from build123d import *

# Parameters (mm, degrees)
F0_R           = 50.8
F1_DEPTH       = 6.35
F3_R           = 25.4
F1_FACE_R      = 50.8
F6_D           = 17.4625
F6_CBORE_D     = 30.1625
F6_CBORE_DEPTH = 19.05


with BuildPart() as f1:
    # F0 (on Top) → F1 (new body)
    with BuildSketch(Plane.XY):
        Circle(F0_R)
    extrude(amount=F1_DEPTH)

    # F3 (on offset) → F4 section 0
    with BuildSketch(Plane.XY.offset(25.4)):
        Circle(F3_R)
    # F1_face (on face) → F4 section 1
    with BuildSketch(Plane.XY.offset(6.35)):
        Circle(F1_FACE_R)
    loft()

    # F6 (through all)
    with Locations(Plane(origin=(0, 0, 0), x_dir=(1, 0, 0), z_dir=(0, 0, -1))):
        with Locations((0, 0)):
            CounterBoreHole(F6_D / 2, F6_CBORE_D / 2, F6_CBORE_DEPTH)


solid = f1.part
CAD build for the part. Positions are in the model's coordinates, mm. A direction names the side the tool comes from. Coordinates: 2 decimals unless noted, no trailing zeros. Loops run counter-clockwise (first coordinate to the right, second up) from the corner with the lowest first, then second, coordinate; pieces in that order, holes last. Notation, with made-up numbers: (62, -3.75) - (89, -3.75) arc R34 cw to (89, 33.25) - close; hole circle Ø3 at (-13.5, -34). An arc over 180 degrees is marked (long way). Write item = value, one per line. Start each with the question number.
Q1. Cut at A-A, the plane x = 0. List the corners of the cut face in (y, z), then the cut area to 3 significant figures.
Q2. Drill centre lines: L1, parallel to Y at x = 0, z = 4.5; L2, parallel to Y at x = 9, z = 12.5; L3, parallel to X at y = -6, z = 24. Where is each one in solid material? Low to high.
Q3. Cut at C-C, the plane z = 15.75. List the corners of the cut face in (x, y).
Q4. Cut at B-B, the plane z = 23.75. List the corners of the cut face in (x, y), then the cut area to 3 significant figures.
Q5. Flat gauge pins, fed straight in: pin 1 Ø1 at (x, z) = (22, 3) entering from -Y; pin 2 Ø3 at (y, z) = (17.5, 8.5) entering from +X; pin 3 Ø10 at (x, z) = (19, 8) entering from +Y. Where does each tip first touch, or does it go through?
Q6. Which spindle directions (+Z, -Z, +X, -X, +Y, -Y) get a long thin tool onto all of the face, cutting with end or side? Do faces 4 (the flat face through (6.5, 6.5, 19.05)), 5 (the flat face through (11, 0, 25.4)). Say none if no direction does.
Q7. Pull direction Y, two halves, no side cores. Call faces 1 (the cylindrical face through (6.93, 5.31, 22.27)), 2 (the cylindrical face through (-11.012, -49.592, 3.131)), 3 (the flat face through (11, 12, 0)): pulls with the +Y half, pulls with the -Y half, needs draft (parallel to the pull), parting line crosses it, or undercut.
Computed:
q1.outline = (-50.8, 0) - (-15.08, 0) - (-15.08, 19.05) - (-8.73, 19.05) - (-8.73, 25.4) - (-25.4, 25.4) - (-50.8, 6.35) - close; (8.73, 19.05) - (15.08, 19.05) - (15.08, 0) - (50.8, 0) - (50.8, 6.35) - (25.4, 25.4) - (8.73, 25.4) - close
q1.area = 1,410 mm²
q2.L1 = -50.8 to -15.08, 15.08 to 50.8
q2.L2 = -41.64 to -12.1, 12.1 to 41.64
q2.L3 = -26.6 to -6.34, 6.34 to 26.6
q3.outline = circle Ø76.53 at (0, 0); hole circle Ø30.16 at (0, 0)
q4.outline = circle Ø55.2 at (0, 0); hole circle Ø17.46 at (0, 0)
q4.area = 2,150 mm²
q5.pin_1 = -46.03
q5.pin_2 = 46.84
q5.pin_3 = 48.75
q6.face_4 = -Z
q6.face_5 = +Z, +X, -X, +Y, -Y
q7.face_1 = undercut
q7.face_2 = parting line crosses it
q7.face_3 = needs draft
